Here's how the part is built. I have some questions about the finished solid (model axes, mm). Coordinates: 2 decimals unless noted, no trailing zeros. Write each loop counter-clockwise with the first axis right and the second up, starting at its lowest first coordinate (ties: lowest second). Pieces come first, ordered by that corner, then holes.
from build123d import *

# Parameters (mm, degrees)
SKETCH1_R           = 101.6
BOSS_EXTRUDE1_DEPTH = 5.55625


with BuildPart() as part:
    # Sketch1 → Boss-Extrude1 (new, symmetric)
    with BuildSketch(Plane(origin=(0, 0, 0), x_dir=(0, 0, -1), z_dir=(1, 0, 0))):
        Circle(SKETCH1_R)
        with BuildLine():
            Line((-2.5, 6.538348415), (-2.5, 8.9))
            Line((-2.5, 8.9), (2.5, 8.9))
            Line((2.5, 8.9), (2.5, 6.538348415))
            ThreePointArc((2.5, 6.538348415), (0, -7), (-2.5, 6.538348415))
        make_face(mode=Mode.SUBTRACT)
    extrude(amount=BOSS_EXTRUDE1_DEPTH, both=True)


solid = part.part
1. If I drill on line 1 (Z direction, x = 1.25, y = 6); line 2 (Y direction, x = 3, z = 59); line 3 (Z direction, x = 4.25, y = 83), over which ranges is the centre line in solid material (lowest first)?
2. I want a section at D-D (y = 74.5). List the corners of the cut face in (x, z) for me, then the cut area to 3 significant figures.
3. For pin 1 Ø1.9 at (x, y) = (2, 7.5) entering from +Z; pin 2 Ø1.5 at (x, z) = (4, 73.5) entering from -Y; pin 3 Ø3 at (x, y) = (1.5, -30.5) entering from +Z, each with a flat end and sliding along its axis, tell me the tip position at first contact or that it passes through.
4. I want a section at A-A (z = 0). List the corners of the cut face in (x, y) for me.
5. I want a section at B-B (y = 0). List the corners of the cut face in (x, z) for me.
6. I want a section at C-C (x = 2.5). List the corners of the cut face in (y, z) for me.
7. Thinking about a two-plate mould opening in Z: for faces 1 (the face through (5.556, 1, -21)), 2 (the face through (0.078, -99.184, 22.025)), 3 (the face through (0, 8.9, 0)), which applies, pulls with the +Z half, pulls with the -Z half, needs draft (parallel to the pull), parting line crosses it, or undercut?
Response values:
1. line 1: z = -101.42 to -3.61, 3.61 to 101.42
1. line 2: y = -82.71 to 82.71
1. line 3: z = -58.6 to 58.6
2. outline: (-5.56, -69.08) - (5.56, -69.08) - (5.56, 69.08) - (-5.56, 69.08) - close
2. area: 1,540 mm2
3. pin 1: stops at z = 101.39
3. pin 2: stops at y = -70.92
3. pin 3: stops at z = 97.37
4. outline: (-5.56, -101.6) - (5.56, -101.6) - (5.56, -7) - (-5.56, -7) - close; (-5.56, 8.9) - (5.56, 8.9) - (5.56, 101.6) - (-5.56, 101.6) - close
5. outline: (-5.56, -101.6) - (5.56, -101.6) - (5.56, -7) - (-5.56, -7) - close; (-5.56, 7) - (5.56, 7) - (5.56, 101.6) - (-5.56, 101.6) - close
6. outline: circle Ø203.2 at (0, 0); hole (6.54, -2.5) - (8.9, -2.5) - (8.9, 2.5) - (6.54, 2.5) arc R7 ccw (long way) to start
7. face 1: needs draft
7. face 2: parting line crosses it
7. face 3: undercut
